from build123d import *

# Parameters (mm, degrees)
SKETCH1_W           = 20.6
SKETCH1_H           = 7
BOSS_EXTRUDE1_DEPTH = 1.5
SKETCH2_W           = 20.6
SKETCH2_H           = 7
SKETCH2_W_2         = 18.6
SKETCH2_H_2         = 5
BOSS_EXTRUDE2_DEPTH = 2
SKETCH3_W           = 1
SKETCH3_H           = 2
CUT_EXTRUDE1_DEPTH  = 13.935996289
BOSS_EXTRUDE3_DEPTH = 6
CUT_EXTRUDE3_DEPTH  = 12.63106466
BOSS_EXTRUDE4_DEPTH = 3
SKETCH5_R           = 0.8
SKETCH5_R_2         = 0.4
CUT_EXTRUDE2_DEPTH  = 12.63106466


with BuildPart() as part:
    # Sketch1 → Boss-Extrude1 (new body)
    with BuildSketch(Plane(origin=(0, 0, 0), x_dir=(1, 0, 0), z_dir=(0, 1, 0))):
        Rectangle(SKETCH1_W, SKETCH1_H)
    extrude(amount=BOSS_EXTRUDE1_DEPTH)

    # Sketch2 → Boss-Extrude2 (add)
    with BuildSketch(Plane(origin=(0, 1.5, 0), x_dir=(1, 0, 0), z_dir=(0, 1, 0))):
        Rectangle(SKETCH2_W, SKETCH2_H)
        Rectangle(SKETCH2_W_2, SKETCH2_H_2, mode=Mode.SUBTRACT)
    extrude(amount=BOSS_EXTRUDE2_DEPTH)

    # Sketch3 → Cut-Extrude1 (cut, through all)
    with BuildSketch(Plane.XY.offset(3.5)):
        with Locations((3.5, 2.5)):
            Rectangle(SKETCH3_W, SKETCH3_H)
        with Locations((-3.5, 2.5)):
            Rectangle(SKETCH3_W, SKETCH3_H)
    extrude(amount=-CUT_EXTRUDE1_DEPTH, mode=Mode.SUBTRACT)

    # Sketch4 → Boss-Extrude3 (add)
    with BuildSketch(Plane.ZY.offset(3)):
        Polygon((-2.5, 4.5), (-2.25, 4.5), (-2.25, 4.75), (-2.75, 5.616025404), (-3.5, 5.616025404), (-3.5, 3.87609405), (-3.5, 3.5), (-2.5, 3.5), align=None)
    boss_extrude3 = extrude(amount=-BOSS_EXTRUDE3_DEPTH)

    # Mirror1: Boss-Extrude3 across plane
    add(boss_extrude3.mirror(Plane.XY))

    # Sketch6 → Cut-Extrude3 (cut, through all)
    with BuildSketch(Plane(origin=(0, 1.5, 0), x_dir=(1, 0, 0), z_dir=(0, 1, 0))):
        with BuildLine():
            Line((8.35, 1.27), (8.35, -1.27))
            ThreePointArc((8.35, -1.27), (7.6, -2.02), (6.85, -1.27))
            Line((6.85, -1.27), (6.85, 1.27))
            ThreePointArc((6.85, 1.27), (7.6, 2.02), (8.35, 1.27))
        make_face()
        with BuildLine():
            Line((-5.25, 0.52), (-5.25, -0.52))
            ThreePointArc((-5.25, -0.52), (-7, -2.27), (-8.75, -0.52))
            Line((-8.75, -0.52), (-8.75, 0.52))
            ThreePointArc((-8.75, 0.52), (-7, 2.27), (-5.25, 0.52))
        make_face()
    extrude(amount=-CUT_EXTRUDE3_DEPTH, mode=Mode.SUBTRACT)

    # Sketch8 → Boss-Extrude4 (add, symmetric)
    with BuildSketch(Plane(origin=(0, 0, 0), x_dir=(0, 0, -1), z_dir=(1, 0, 0))):
        with BuildLine():
            Line((-3.5, 0), (-3.098076211, -1.5))
            Line((-3.098076211, -1.5), (-2.145, -1.5))
            ThreePointArc((-2.145, -1.5), (-1.27, -0.625), (-0.395, -1.5))
            Line((-0.395, -1.5), (0.87, -1.5))
            Line((0.87, -1.5), (0.87, -1))
            ThreePointArc((0.87, -1), (1.27, -0.6), (1.67, -1))
            Line((1.67, -1), (3.232050808, -1))
            Line((3.232050808, -1), (3.5, 0))
            Line((3.5, 0), (-3.5, 0))
        make_face()
    extrude(amount=BOSS_EXTRUDE4_DEPTH, both=True)

    # Sketch5 → Cut-Extrude2 (cut, through all)
    with BuildSketch(Plane(origin=(0, 1.5, 0), x_dir=(1, 0, 0), z_dir=(0, 1, 0))):
        with Locations(Location((0, 0, 0), (0, 0, 270))):
            Circle(SKETCH5_R)
        with Locations(Location((8.95, -2, 0), (0, 0, 270))):
            Circle(SKETCH5_R_2)
    extrude(amount=-CUT_EXTRUDE2_DEPTH, mode=Mode.SUBTRACT)


solid = part.part
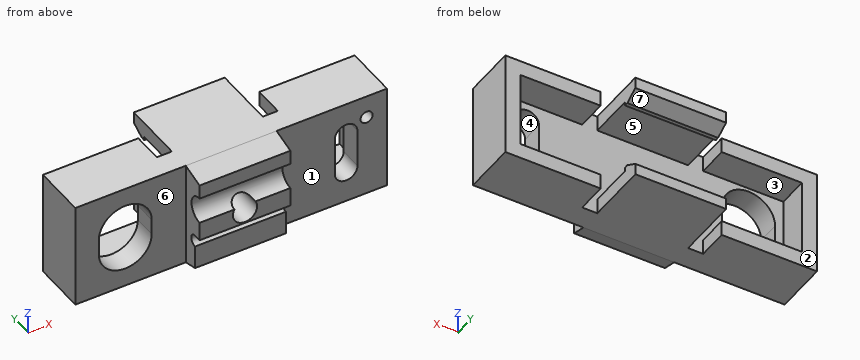
Geometry: final body of the model. Coordinates: model frame, mm. Face numbers are marked on the shaded views. A direction names the side the tool comes from. Give positions to 0.01 mm unless a question says otherwise; leave off trailing zeros. Loops run counter-clockwise (first coordinate to the right, second up) from the corner with the lowest first, then second, coordinate; pieces in that order, holes last. Notation, with made-up numbers: (71.5, -30) - (97.5, -30) arc R14 cw to (97.5, -23) - close; hole circle Ø5 at (87.5, 52). An arc over 180 degrees is marked (long way). Answer as CSV lines item,"result". Start each with the question number.
1. Reachability of the marked faces 1, 2 and 3 from +Z, -Z, +X, -X, +Y, -Y: full face, straight path, thin tool, end or side. Return the list, or none.
2. Pin query (flat end, axial travel): P1, Ø0.6, axis at x = 0.5, y = -1, coming from the -Z side; P2, Ø2, axis at x = 2, z = 1, coming from the +Y side. Return the tip coordinate at first contact, or that it passes through.
3. Section B-B, the plane z = 0. Return loops of the section in (x, y).
4. Draft query along Y for the marked faces 4, 5, 6 and 7. Return one class per face: released by +Y, released by -Y, zero draft, split by the parting line, or undercut.
5. Section C-C, the plane x = 7.6. Return loops of the section in (y, z), plus the area to 3 significant figures.
6. Section A-A, the plane y = 2.5. Return loops of the section in (x, z), plus the area to 3 significant figures.
7. Section D-D, the plane x = -5. Return loops of the section in (y, z), plus the area to 3 significant figures.
8. Ray query, L1, parallel to Z at x = 2.5, y = 2.25; L2, parallel to Z at x = 8.95, y = 0.35; L3, parallel to X at y = 1, z = 1.5. Return the intervals inside material, ascending.
Answers:
1,face 1,"+Z, -Z, +X, -Y"
1,face 2,"+Z, -Z, -X, +Y"
1,face 3,"+Y"
2,P1,"stops at z = -3.31"
2,P2,"stops at y = 1.5"
3,outline,"(-10.3, 0) - (-8.75, 0) - (-8.75, 1.5) - (-9.3, 1.5) - (-9.3, 3.5) - (-10.3, 3.5) - close; (-5.25, 0) - (-3, 0) - (-3, -1.5) - (-0.8, -1.5) - (-0.8, 1.5) - (-5.25, 1.5) - close; (0.8, -1.5) - (3, -1.5) - (3, 0) - (6.85, 0) - (6.85, 1.5) - (0.8, 1.5) - close; (8.35, 0) - (10.3, 0) - (10.3, 3.5) - (9.3, 3.5) - (9.3, 1.5) - (8.35, 1.5) - close"
4,face 4,"zero draft"
4,face 5,"undercut"
4,face 6,"released by -Y"
4,face 7,"released by +Y"
5,outline,"(0, -3.5) - (3.5, -3.5) - (3.5, -2.5) - (1.5, -2.5) - (1.5, -2.02) - (0, -2.02) - close; (0, 2.02) - (1.5, 2.02) - (1.5, 2.5) - (3.5, 2.5) - (3.5, 3.5) - (0, 3.5) - close"
5,area,"8.44 mm2"
6,outline,"(-10.3, -3.5) - (-4, -3.5) - (-4, -2.5) - (-9.3, -2.5) - (-9.3, 2.5) - (-4, 2.5) - (-4, 3.5) - (-10.3, 3.5) - close; (-3, -3.5) - (3, -3.5) - (3, -2.5) - (-3, -2.5) - close; (-3, 2.5) - (3, 2.5) - (3, 3.5) - (-3, 3.5) - close; (4, -3.5) - (10.3, -3.5) - (10.3, 3.5) - (4, 3.5) - (4, 2.5) - (9.3, 2.5) - (9.3, -2.5) - (4, -2.5) - close"
6,area,"47.2 mm2"
7,outline,"(0, -3.5) - (3.5, -3.5) - (3.5, -2.5) - (1.5, -2.5) - (1.5, 2.5) - (3.5, 2.5) - (3.5, 3.5) - (0, 3.5) - close"
7,area,"14.5 mm2"
8,L1,"z = -3.5 to -2.5, 2.5 to 3.5"
8,L2,"z = -3.5 to 1.6, 2.4 to 3.5"
8,L3,"x = -10.3 to -8.45, -5.55 to 6.89, 8.31 to 10.3"
